Part model, mm, in its own coordinate system. Face numbers are marked on the shaded views. A direction names the side the tool comes from. Coordinates: 2 decimals unless noted, no trailing zeros. Loops run counter-clockwise (first coordinate to the right, second up) from the corner with the lowest first, then second, coordinate; pieces in that order, holes last. Notation, with made-up numbers: (10, 56) - (57, 56) arc R12 ccw to (57, 69) - close; hole circle Ø9 at (78.5, 78). An arc over 180 degrees is marked (long way). Use a Markdown table: item, result. Add a question column.
1. Wall check: probe 1 along X at (y, z) = (8.75, 2); probe 2 along Y at (x, z) = (9.5, 8.5); probe 3 along X at (y, z) = (2.75, 6.25). Give the ranges that are in metal, low to high. Write a range as [from, to].
2. Pull direction X, two halves, no side cores. Call the marked faces 6, 7 and 8: pulls with the +X half, pulls with the -X half, needs draft (parallel to the pull), parting line crosses it, or undercut.
3. Band-saw the part on D-D, the plane x = 17.25. Give the cut face in (y, z).
4. Band-saw the part on A-A, the plane y = 9.5. Give the cut face in (x, z).
5. Band-saw the part on C-C, the plane z = 9.25. Give the cut face in (x, y), plus the area to 3 significant figures.
6. Band-saw the part on B-B, the plane y = 1. Count the separate pieces of the cut face and the enclosed holes in it, plus the area to 3 significant figures.
7. Drop flat-ended pins along their axis: pin 1 (5 mm diameter, centred on x = 18.5, z = 6, fed in from +Y); pin 2 (0.7 mm diameter, centred on x = -1, y = 1, fed in from +Z); pin 3 (4 mm diameter, centred on y = 7.5, z = 6.5, fed in from -X). Give the stop position or say it passes through.
8. 3-axis set-ups, long thin cutter, end or side, ignore diameter. For the marked faces 1, 2, 3, 4 and 5: which of +Z, -Z, +X, -X, +Y, -Y reach the whole face in a straight line?
Autodesk Inventor part; units mm, degrees
ref_plane "YZ Plane" through (0, 0, 0) normal (1, 0, 0) x (0, 1, 0)
ref_plane "XZ Plane" through (0, 0, 0) normal (0, 1, 0) x (-1, 0, 0)
ref_plane "XY Plane" through (0, 0, 0) normal (0, 0, 1) x (1, 0, 0)
sketch "Sketch1" plane through (0, 0, 0) normal (0, 0, 1) x (1, 0, 0)
  line L0 (0, 2.9972) -> (0, 11.5062)
  line L1 (0, 11.5062) -> (15.0114, 11.5062)
  line L2 (15.0114, 11.5062) -> (15.0114, 2.9972)
  line L3 (13.5001, 0) -> (13.5001, 9.9949)
  line L4 (13.5001, 9.9949) -> (1.5113, 9.9949)
  line L5 (1.5113, 9.9949) -> (1.5113, 0)
  line L6 (15.0114, 2.9972) -> (20.8026, 2.9972)
  line L7 (20.8026, 2.9972) -> (20.8026, 0)
  line L8 (20.8026, 0) -> (15.0113, 0)
  line L9 (15.0113, 0) -> (13.5001, 0)
  line L10 (0, 0) -> (-5.7912, 0)
  line L11 (-5.7912, 2.9972) -> (0, 2.9972)
  line L12 (0, 0) -> (1.5113, 0)
  line L13 (-5.7912, 2.9972) -> (-5.7912, 0)
  dimension "d0" = 11.5062
  dimension "d2" = 15.0114
  dimension "d3" = 11.9888
  dimension "d4" = 0
  dimension "d5" = 0
  dimension "d6" = 0
  dimension "d7" = 5.7912
  dimension "d8" = 5.7912
  dimension "d9" = 2.9972
  dimension "d10" = 2.9972
extrude "Extrusion1" add sketch "Sketch1" along normal blind 11.5062
sketch "Sketch2" plane through (0, 0, 11.5062) normal (0, 0, 1) x (1, 0, 0)
  line L0 (15.0114, 2.9972) -> (20.8026, 2.9972)
  line L1 (20.8026, 2.9972) -> (20.8026, 0)
  line L2 (20.8026, 0) -> (15.0114, 0)
  line L3 (15.0114, 0) -> (15.0114, 2.9972)
  line L4 (0, 2.9972) -> (-5.7912, 2.9972)
  line L5 (-5.7912, 2.9972) -> (-5.7912, 0)
  line L6 (-5.7912, 0) -> (0, 0)
  line L7 (0, 0) -> (0, 2.9972)
  point P0 (0, 0)
extrude "Extrusion2" cut sketch "Sketch2" against normal blind 2.9972
sketch "Sketch3" plane through (15.0114, 2.9972, 0) normal (0, 1, 0) x (1, 0, 0)
  line L0 (0, 0) -> (0, -8.509)
  arc A0 (1.4999, -5.3467) -> (1.4325, -3.1643) centre (1.4986, -4.2545) ccw
  arc A1 (-16.51, -3.1604) -> (-16.51, -5.3486) centre (-16.51, -4.2545) ccw
  line L1 (-15.0114, 0) -> (-15.0114, -11.5062)
  line L2 (-16.51, -3.1604) -> (-15.0114, -3.1604)
  line L3 (-15.0114, -3.1604) -> (-15.0114, -5.3486)
  line L4 (-15.0114, -5.3486) -> (-16.51, -5.3486)
  line L5 (1.4325, -3.1643) -> (0, -3.1643)
  line L6 (0, -3.1643) -> (0, -5.3486)
  line L7 (0, -5.3486) -> (1.4999, -5.3467)
  dimension "d15" = 2.1844
  dimension "d17" = 1.4986
  dimension "d18" = 1.4986
extrude "Extrusion3" cut sketch "Sketch3" against normal blind 50.8
fillet "Fillet1" radius 4.2545 4 edges at (20.8026, 1.4986, 8.509) (20.8026, 1.4986, 0) (-5.7912, 1.4986, 8.509) (-5.7912, 1.4986, 0)
fillet "Fillet2" radius 1.27 6 edges at (0, 2.9972, 1.5802) (0, 2.9972, 6.9288) (0, 11.5062, 5.7531) (15.0114, 11.5062, 5.7531) (15.0114, 2.9972, 1.5822) (15.0114, 2.9972, 6.9288)
properties part number "Mount_Motor" material "Nylon 6/6"
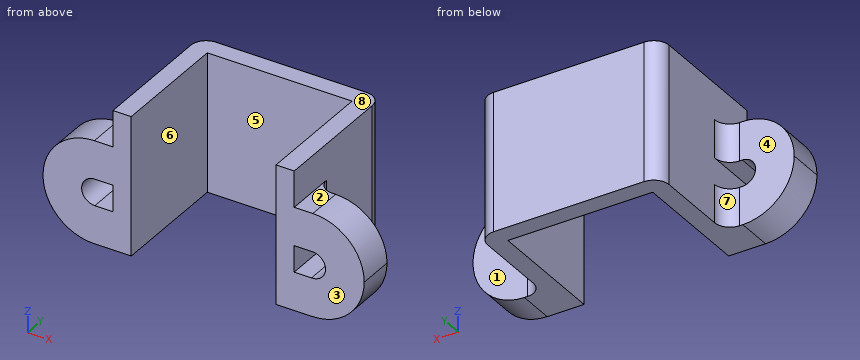
Geometry check:
| question | item | result |
|---|---|---|
| 1 | probe 1 | x = [0, 1.51], [13.5, 15.01] |
| 1 | probe 2 | y = [9.99, 11.51] |
| 1 | probe 3 | x = [-5.29, 1.51], [13.5, 20.31] |
| 2 | face 6 | undercut |
| 2 | face 7 | pulls with the -X half |
| 2 | face 8 | needs draft |
| 3 | outline | (0, 0.06) - (3, 0.06) - (3, 3.45) - (0, 3.45) - close; (0, 5.06) - (3, 5.06) - (3, 8.45) - (0, 8.45) - close |
| 4 | outline | (0, 0) - (1.51, 0) - (1.51, 11.51) - (0, 11.51) - close; (13.5, 0) - (15.01, 0) - (15.01, 11.51) - (13.5, 11.51) - close |
| 5 | outline | (0, 0) - (1.51, 0) - (1.51, 9.99) - (13.5, 9.99) - (13.5, 0) - (15.01, 0) - (15.01, 10.24) arc R1.27 ccw to (13.74, 11.51) - (1.27, 11.51) arc R1.27 ccw to (0, 10.24) - close |
| 5 | area | 52.2 mm^2 |
| 6 | separate pieces | 2 |
| 6 | enclosed holes | 2 |
| 6 | area | 107 mm^2 |
| 7 | pin 1 | stops at y = 3.03 |
| 7 | pin 2 | stops at z = 8.51 |
| 7 | pin 3 | stops at x = 0 |
| 8 | face 1 | +Z, -Z, +X, +Y |
| 8 | face 2 | +Z, +X, +Y, -Y |
| 8 | face 3 | +Z, -Z, +X, -X, -Y |
| 8 | face 4 | +Z, -Z, -X, +Y |
| 8 | face 5 | +Z, -Z, -Y |
